Verification items for the finished model (mm, model axes). Give positions to 0.01 mm unless a question says otherwise; leave off trailing zeros. Loops run counter-clockwise (first coordinate to the right, second up) from the corner with the lowest first, then second, coordinate; pieces in that order, holes last. Notation, with made-up numbers: (7.25, 81) -> (64.25, 81) arc R21 cw to (64.25, 111) -> close; hole circle Ø9 at (58.5, 23.25). An arc over 180 degrees is marked (long way). Answer in a Markdown table with one row per item. Add a question column.
Q1. Section check B-B on z = -92. Enter the section's corners in (x, y).
Q2. Section check A-A on x = 98.5. Enter the section's corners in (y, z).
Q3. Gauge pin test, flat ends, axial feed: P1, Ø1.5, axis at x = -3.5, y = 7.5, coming from the +Z side; P2, Ø5, axis at x = -94, y = 8.5, coming from the +Z side; P3, Ø2, axis at y = 8, z = -81.5, coming from the -X side. Record the tip position at first contact, or that the pin passes through.
Q4. Section check C-C on y = 10.5. Enter the section's corners in (x, z) (3 decimals), and give its area (3 significant figures).
Q5. Material ranges on probe 1 along Z at (x, y) = (1.5, 9.25) (3 decimals); probe 2 along X at (y, z) = (9.5, -17.5); probe 3 along X at (y, z) = (12, 41.5), recorded low to high.
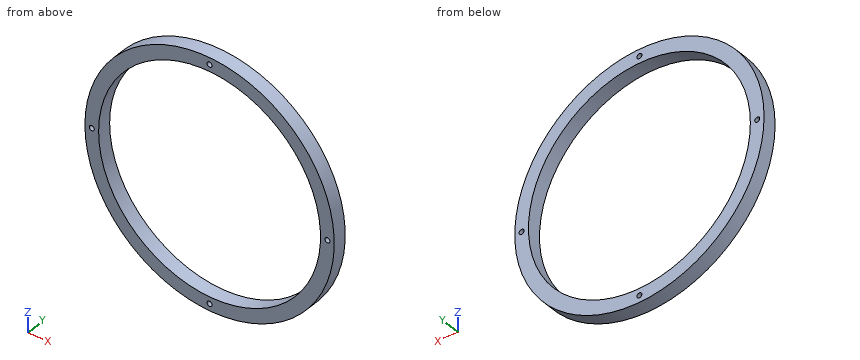
Autodesk Inventor part; units mm, degrees
ref_plane "YZ Plane" through (0, 0, 0) normal (1, 0, 0) x (0, 1, 0)
ref_plane "XZ Plane" through (0, 0, 0) normal (0, 1, 0) x (-1, 0, 0)
ref_plane "XY Plane" through (0, 0, 0) normal (0, 0, 1) x (1, 0, 0)
sketch "Sketch1" plane through (0, 0, 0) normal (0, 1, 0) x (-1, 0, 0)
  circle A0 centre (0, 0) radius 125
  circle A1 centre (0, 0) radius 111.25
  dimension "d0" = 250
  dimension "d1" = 222.5
extrude "Extrusion1" add sketch "Sketch1" along normal blind 14
sketch "Sketch2" plane through (0, 14, 0) normal (0, 1, 0) x (1, 0, 0)
  circle A0 centre (0, 0) radius 118.125
  point P0 (0, 118.125)
  dimension "d4" = 236.25
hole "Hole1" at (0, 14, -118.125) direction (0, -1, 0) diameter 5 end through all
pattern_circular "Circular Pattern1" count 4 over 360 about axis through (0, -10, 0) along (0, 1, 0) of "Hole1"
sketch "Sketch3" plane through (0, 14, 0) normal (0, 1, 0) x (1, 0, 0)
  point P0 (0, 0)
properties part number "BearingTableGear"
Taken from the geometry:
| question | item | result |
|---|---|---|
| 1 | outline | (-84.62, 0) -> (-62.55, 0) -> (-62.55, 14) -> (-84.62, 14) -> close; (62.55, 0) -> (84.62, 0) -> (84.62, 14) -> (62.55, 14) -> close |
| 2 | outline | (0, -76.96) -> (14, -76.96) -> (14, -51.71) -> (0, -51.71) -> close; (0, 51.71) -> (14, 51.71) -> (14, 76.96) -> (0, 76.96) -> close |
| 3 | P1 | stops at z = 124.97 |
| 3 | P2 | stops at z = 85.16 |
| 3 | P3 | stops at x = -95.63 |
| 4 | outline | circle Ø250 at (0, 0); hole circle Ø5 at (-118.125, 0); hole circle Ø222.5 at (0, 0); hole circle Ø5 at (0, -118.125); hole circle Ø5 at (0, 118.125); hole circle Ø5 at (118.125, 0) |
| 4 | area | 10,100 mm² |
| 5 | probe 1 | z = -124.991 to -120.125, -116.125 to -111.24, 111.24 to 116.125, 120.125 to 124.991 |
| 5 | probe 2 | x = -123.77 to -109.86, 109.86 to 123.77 |
| 5 | probe 3 | x = -117.91 to -103.22, 103.22 to 117.91 |
